```python
from build123d import *

# Parameters (mm, degrees)
SKETCH2_R           = 2.1
BOSS_EXTRUDE1_DEPTH = 1.2
CUT_EXTRUDE1_DEPTH  = 1.5
SKETCH4_R           = 2.1
BOSS_EXTRUDE3_DEPTH = 1.2
CUT_EXTRUDE2_DEPTH  = 1.5


with BuildPart() as part:
    # Sketch2 → Boss-Extrude1 (new body)
    with BuildSketch(Plane(origin=(0, 0, 0), x_dir=(1, 0, 0), z_dir=(0, 1, 0))):
        Polygon((39.4127274, 50.640295112), (39.4127274, 0.640295112), (-45.5872726, 0.640295112), (-80.5872726, 50.640295112), align=None)
        with Locations((22.381300815, 25.64100497)):
            Circle(SKETCH2_R, mode=Mode.SUBTRACT)
    extrude(amount=BOSS_EXTRUDE1_DEPTH)

    # Sketch3 → Cut-Extrude1 (cut)
    with BuildSketch(Plane(origin=(0, 1.2, 0), x_dir=(1, 0, 0), z_dir=(0, 1, 0))):
        Polygon((39.4127274, 40.640295112), (-30.5872726, 40.640295112), (-50.5872726, 50.640295112), (39.4127274, 50.640295112), align=None)
    extrude(amount=-CUT_EXTRUDE1_DEPTH, mode=Mode.SUBTRACT)

    # Sketch4 → Boss-Extrude3 (add)
    with BuildSketch(Plane(origin=(0, 1.2, 0), x_dir=(1, 0, 0), z_dir=(0, 1, 0))):
        Polygon((39.4127274, 0.640295112), (-60.5872726, 0.640295112), (-100.5872726, 60.640295112), (-60.5872726, 60.640295112), (-44.926762529, 45.640295112), (39.4127274, 45.640295112), align=None)
        with Locations((22.381300815, 25.64100497)):
            Circle(SKETCH4_R, mode=Mode.SUBTRACT)
    extrude(amount=-BOSS_EXTRUDE3_DEPTH)

    # Sketch6 → Cut-Extrude2 (cut)
    with BuildSketch(Plane(origin=(0, 1.2, 0), x_dir=(1, 0, 0), z_dir=(0, 1, 0))):
        Polygon((-40.5872726, 45.640295112), (-44.926762529, 45.640295112), (-49.666026343, 50.179671984), align=None)
    extrude(amount=-CUT_EXTRUDE2_DEPTH, mode=Mode.SUBTRACT)


solid = part.part
```
The model under review builds one solid part; all positions refer to its coordinate system, in mm. Round coordinates to 2 decimals unless told otherwise and drop trailing zeros. Loops run counter-clockwise (first coordinate to the right, second up) from the corner with the lowest first, then second, coordinate; pieces in that order, holes last. Notation, with made-up numbers: (-3.75, 27.5) - (7.25, 27.5) arc R24 cw to (7.25, 53.5) - close; hole circle Ø4 at (5, -10.75). An arc over 180 degrees is marked (long way). Use a Markdown table: item, result. Add a question column.
Q1. Add section B-B (x = -2). State the section outline as (y, z) points, plus the area to 3 significant figures.
Q2. The part is to be moulded in two halves that separate along X. For faces 1 (the face through (-80.307, 0.608, -30.22)), 2 (the face through (-30, 0, -31)), 3 (the face through (23.51, 0.59, -27.41)), say which applies: pulls with the +X half, pulls with the -X half, needs draft (parallel to the pull), parting line crosses it, or undercut.
Q3. Add section C-C (z = -35). State the section outline as (x, y) points, plus the area to 3 significant figures.
Q4. For probe 1 along Z at (x, y) = (-42, 0.25); probe 2 along Z at (x, y) = (-81, 0.7); probe 3 along X at (y, z) = (0.65, -45.5), list the stretches that pass through material, from the lowest coordinate up.
Q5. Insertion check: pin 1 Ø3.5 at (x, z) = (22.38, -25.64) entering from -Y (1 decimal). The pin has a flat end and moves straight along its axis. Give the tip position at first contact, or say it passes through.
Q6. Add section A-A (y = 0.45). State the section outline as (x, z) points.
Worked answers:
| question | item | result |
|---|---|---|
| 1 | outline | (0, -45.64) - (1.2, -45.64) - (1.2, -0.64) - (0, -0.64) - close |
| 1 | area | 54.0 mm² |
| 2 | face 1 | pulls with the -X half |
| 2 | face 2 | needs draft |
| 2 | face 3 | undercut |
| 3 | outline | (-83.49, 0) - (39.41, 0) - (39.41, 1.2) - (-83.49, 1.2) - close |
| 3 | area | 147 mm² |
| 4 | probe 1 | -45.64 to -0.64 |
| 4 | probe 2 | -60.64 to -31.26 |
| 4 | probe 3 | -90.49 to 39.41 |
| 5 | pin 1 | through |
| 6 | outline | (-100.59, -60.64) - (-60.59, -60.64) - (-44.93, -45.64) - (39.41, -45.64) - (39.41, -0.64) - (-60.59, -0.64) - close; hole circle Ø4.2 at (22.38, -25.64) |
